```python
from build123d import *

# Parameters (mm, degrees)
F2_DEPTH = 74.422
F0_W     = 114.037246
F0_H     = 8.752351
F3_DEPTH = 25.4
F0_W_2   = 114.037238
F0_H_2   = 6.529795
F4_DEPTH = 25.4
F0_W_3   = 114.03723
F0_H_3   = 8.757952
F5_DEPTH = 25.4
F0_H_4   = 7.899019
F6_DEPTH = 25.4


with BuildPart() as f2:
    # F1 (on Right) → F2 (new body, symmetric)
    with BuildSketch(Plane.YZ):
        Polygon((42.566895, 0), (-76.200001, 0), (-76.200001, -39.413795), align=None)
    extrude(amount=F2_DEPTH, both=True)

    # F0 (on Top) → F3 (cut)
    with BuildSketch(Plane.XY):
        with Locations((0, -26.185142)):
            Rectangle(F0_W, F0_H)
    extrude(amount=-F3_DEPTH, mode=Mode.SUBTRACT)

    # F0 (on Top) → F4 (cut)
    with BuildSketch(Plane.XY):
        with Locations((0, -38.776483)):
            Rectangle(F0_W_2, F0_H_2)
    extrude(amount=-F4_DEPTH, mode=Mode.SUBTRACT)

    # F0 (on Top) → F5 (cut)
    with BuildSketch(Plane.XY):
        with Locations((0, -54.135197)):
            Rectangle(F0_W_3, F0_H_3)
    extrude(amount=-F5_DEPTH, mode=Mode.SUBTRACT)

    # F0 (on Top) → F6 (cut)
    with BuildSketch(Plane.XY):
        with Locations((0, -67.32359)):
            Rectangle(F0_W, F0_H_4)
    extrude(amount=-F6_DEPTH, mode=Mode.SUBTRACT)


solid = f2.part
```
Build history of the part. All positions in model axes, mm. A direction names the side the tool comes from. Round coordinates to 2 decimals unless told otherwise and drop trailing zeros. Order: outer loops, then holes, each group sorted by start corner. A loop starts at its lowest first (then second) coordinate and runs counter-clockwise, first axis right, second up. Notation, with made-up numbers: (55, 74.5) - (88, 74.5) arc R24 cw to (88, 89.5) - close; hole circle Ø10 at (89, -10). An arc over 180 degrees is marked (long way). Use a Markdown table: item, result.
1) Pull direction Y, two halves, no side cores. Call faces 1 (the face through (1, -76.2, -19)), 2 (the face through (-74.422, -31, -15)), 3 (the face through (57.019, -54, -13)): pulls with the +Y half, pulls with the -Y half, needs draft (parallel to the pull), parting line crosses it, or undercut.
Recorded:
| item | result |
|---|---|
| face 1 | pulls with the -Y half |
| face 2 | needs draft |
| face 3 | undercut |
2) Saw through at A-A on x = 19.5. Write the cut outline in (y, z).
Recorded:
| item | result |
|---|---|
| outline | (-76.2, -39.41) - (-30.56, -24.27) - (-30.56, 0) - (-35.51, 0) - (-35.51, -25.4) - (-42.04, -25.4) - (-42.04, 0) - (-49.76, 0) - (-49.76, -25.4) - (-58.51, -25.4) - (-58.51, 0) - (-63.37, 0) - (-63.37, -25.4) - (-71.27, -25.4) - (-71.27, 0) - (-76.2, 0) - close; (-21.81, -21.36) - (42.57, 0) - (-21.81, 0) - close |
3) Flat gauge pins, fed straight in: pin 1 Ø2.5 at (x, y) = (-2.5, -67) entering from +Z; pin 2 Ø7 at (x, y) = (-27.5, -38.5) entering from +Z. Where does each tip first touch, or does it go through?
Recorded:
| item | result |
|---|---|
| pin 1 | stops at z = -25.4 |
| pin 2 | stops at z = 0 |
4) Saw through at B-B on y = -26. Write the cut outline in (x, z), and give its area (3 significant figures).
Recorded:
| item | result |
|---|---|
| outline | (-74.42, -22.75) - (-57.02, -22.75) - (-57.02, 0) - (-74.42, 0) - close; (57.02, -22.75) - (74.42, -22.75) - (74.42, 0) - (57.02, 0) - close |
| area | 792 mm² |
5) Saw through at D-D on y = -40. Write the cut outline in (x, z), and give its area (3 significant figures).
Recorded:
| item | result |
|---|---|
| outline | (-74.42, -27.4) - (74.42, -27.4) - (74.42, 0) - (57.02, 0) - (57.02, -25.4) - (-57.02, -25.4) - (-57.02, 0) - (-74.42, 0) - close |
| area | 1,180 mm² |
6) Wall check: L1, parallel to X at y = -71, z = -24.5; L2, parallel to Z at x = -56, y = -71; L3, parallel to Z at x = -4, y = -56. Give the ranges that are in metal, low to high.
Recorded:
| item | result |
|---|---|
| L1 | x = -74.42 to -57.02, 57.02 to 74.42 |
| L2 | z = -37.69 to -25.4 |
| L3 | z = -32.71 to -25.4 |
7) Tool access for faces 4 (the face through (-57.019, -26, -12)), 5 (the face through (74.422, -31, -15)), 6 (the face through (-1, -35.512, -13)): list every direction of +Z, -Z, +X, -X, +Y, -Y with a clear straight run to the whole face (end or side of a thin tool).
Recorded:
| item | result |
|---|---|
| face 4 | +Z, -Z |
| face 5 | +Z, -Z, +X, +Y, -Y |
| face 6 | +Z |
8) Saw through at C-C on z = -11. Write the cut outline in (x, y), and give its area (3 significant figures).
Recorded:
| item | result |
|---|---|
| outline | (-74.42, -76.2) - (74.42, -76.2) - (74.42, 9.42) - (-74.42, 9.42) - close; hole (-57.02, -71.27) - (57.02, -71.27) - (57.02, -63.37) - (-57.02, -63.37) - close; hole (-57.02, -58.51) - (57.02, -58.51) - (57.02, -49.76) - (-57.02, -49.76) - close; hole (-57.02, -42.04) - (57.02, -42.04) - (57.02, -35.51) - (-57.02, -35.51) - close; hole (-57.02, -30.56) - (57.02, -30.56) - (57.02, -21.81) - (-57.02, -21.81) - close |
| area | 9,100 mm² |
